Geometry: see drawing. Coordinates: mm, zero at the bounding-box minimum. Round coordinates to 2 decimals unless told otherwise and drop trailing zeros. Order: outer loops, then holes, each group sorted by start corner. A loop starts at its lowest first (then second) coordinate and runs counter-clockwise, first axis right, second up. Notation, with made-up numbers: (-17, 65.5) -> (33, 65.5) arc R11 cw to (33, 74.5) -> close; hole circle Ø2 at (-18.75, 30). An arc over 180 degrees is marked (long way). Put each result on its own line as item: value.
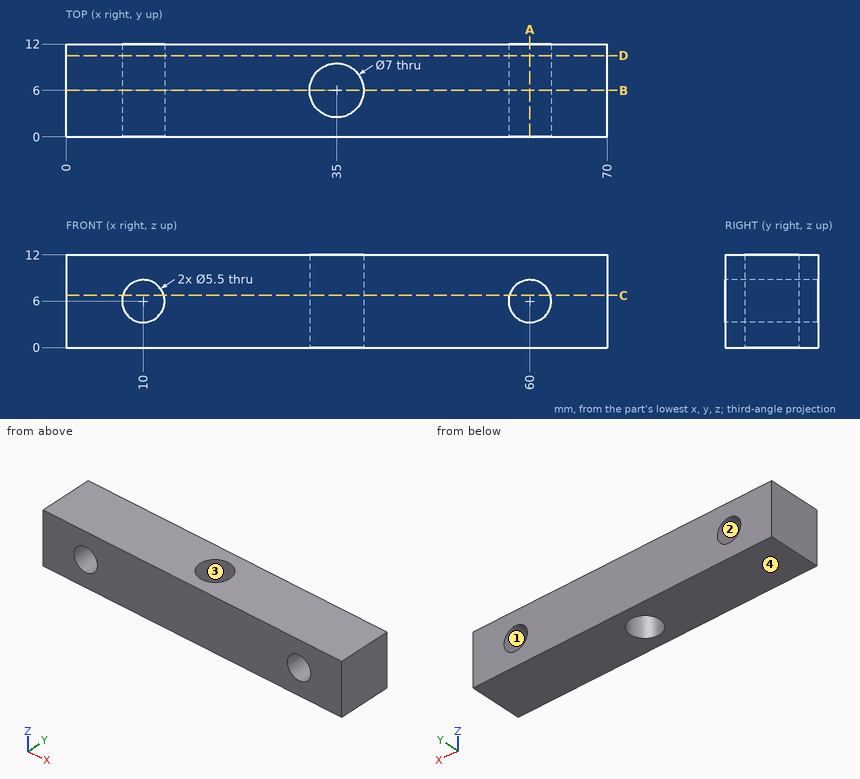
1. Cut plane B-B on y = 6. Return loops of the section in (x, z).
Ans:
outline: (0, 0) -> (31.5, 0) -> (31.5, 12) -> (0, 12) -> close; (38.5, 0) -> (70, 0) -> (70, 12) -> (38.5, 12) -> close; hole circle Ø5.5 at (10, 6); hole circle Ø5.5 at (60, 6)
2. Material intervals for probe 1 along Y at (x, z) = (35, 6); probe 2 along X at (y, z) = (3.75, 5.25); probe 3 along X at (y, z) = (8.5, 7), sorted ascending.
Ans:
probe 1: 0 to 2.5, 9.5 to 12
probe 2: 0 to 7.35, 12.65 to 32.32, 37.68 to 57.35, 62.65 to 70
probe 3: 0 to 7.44, 12.56 to 32.55, 37.45 to 57.44, 62.56 to 70
3. Cut plane C-C on z = 6.75. Return loops of the section in (x, y).
Ans:
outline: (0, 0) -> (7.35, 0) -> (7.35, 12) -> (0, 12) -> close; (12.65, 0) -> (57.35, 0) -> (57.35, 12) -> (12.65, 12) -> close; (62.65, 0) -> (70, 0) -> (70, 12) -> (62.65, 12) -> close; hole circle Ø7 at (35, 6)
4. Draft query along Z for the marked faces 1, 2, 3 and 4. Return one class per face: +Z half, -Z half, draft (parallel to the pull), parting line (faces both ways), or undercut.
Ans:
face 1: undercut
face 2: undercut
face 3: draft
face 4: -Z half
5. Cut plane A-A on x = 60. Return loops of the section in (y, z), and give its area (3 significant figures).
Ans:
outline: (0, 0) -> (12, 0) -> (12, 3.25) -> (0, 3.25) -> close; (0, 8.75) -> (12, 8.75) -> (12, 12) -> (0, 12) -> close
area: 78.0 mm²
6. Cut plane D-D on y = 10.5. Return loops of the section in (x, z).
Ans:
outline: (0, 0) -> (70, 0) -> (70, 12) -> (0, 12) -> close; hole circle Ø5.5 at (10, 6); hole circle Ø5.5 at (60, 6)
